Design review of the part built by this model. Coordinates are the model's own, in mm. A direction names the side the tool comes from. Coordinates: 2 decimals unless noted, no trailing zeros. Loops run counter-clockwise (first coordinate to the right, second up) from the corner with the lowest first, then second, coordinate; pieces in that order, holes last. Notation, with made-up numbers: (2.25, 28.25) - (51.25, 28.25) arc R10 cw to (51.25, 35.25) - close; hole circle Ø7 at (-19, 14.5). An arc over 180 degrees is marked (long way). Answer in a Markdown table with one row per item. Add a question column.
(1) To check wall thickness, follow L1, parallel to X at y = 41, z = 57.5; L2, parallel to X at y = 41, z = 78; L3, parallel to Y at x = 43.5, z = 97. State the ranges of each line that lie inside material, in increasing order. Write a range as [from, to].
(2) For faces 1 (the face through (57, 67, 85)), 2 (the face through (-43.325, 47.12, 64.65)), 3 (the face through (-53, -3, 90)), 4 (the face through (21, 75, 82)), list the 3-axis set-ups (+Z, -Z, +X, -X, +Y, -Y) from which the entire face can be reached by the end or side of a thin tool; tool diameter is ignored.
(3) We need section B-B, the plane x = -25.5. Write out the cut boundary in (y, z).
(4) Clearance check with flat-ended pins moving along their axes: pin 1 (9 mm diameter, centred on y = -81, z = 81.5, fed in from +X); pin 2 (10 mm diameter, centred on x = 21.5, y = -54, fed in from +Z); pin 3 (14.5 mm diameter, centred on x = -46.5, y = 39.5, fed in from +Z). State where each tip first meets the part, or that it passes through.
(5) We need section D-D, the plane z = 96.5. Write out the cut boundary in (x, y).
(6) We need section A-A, the plane y = 41. Write out the cut boundary in (x, z).
(7) We need section C-C, the plane z = 65. Write out the cut boundary in (x, y).
(8) The part is to be moulded in two halves that separate along X. For faces 5 (the face through (42, -78, 30)), 6 (the face through (-6, 100, 54)), 7 (the face through (14.566, 67.605, 89.002)), say which applies: released by +X, released by -X, zero draft, split by the parting line, or undercut.
Autodesk Fusion 360 part; units mm, degrees
sketch "Sketch1" plane through (0, 0, 0) normal (0, 0, 1) x (1, 0, 0)
  line L0 (-75, 100) -> (65, 100)
  line L1 (65, 100) -> (65, -100)
  line L2 (65, -100) -> (-75, -100)
  line L3 (-75, -100) -> (-75, 100)
  line L4 (38.9966, -100) -> (40, -100)
  line L5 (20, -100) -> (65, -55)
  line L6 (-60, -100) -> (-60, -50)
  line L7 (-60, -50) -> (-20, 30)
  line L8 (-20, 30) -> (-20, 60)
  line L9 (-20, 60) -> (50, 60)
  line L10 (50, 60) -> (70, 80)
  line L11 (70, 80) -> (70, 100)
  line L12 (-20, 60) -> (-75, 60)
extrude "Extrude1" add sketch "Sketch1" along normal blind 20 contours L1 L2 L5 L6 L7 L8 L9 L10
extrude "Extrude2" add sketch "Sketch1" along normal blind 40 contours L2 L3 L6 L7 L8 L12
extrude "Extrude3" add sketch "Sketch1" along normal blind 70 contours L0 L1 L3 L9 L10 L12
sketch "Sketch2" plane through (0, 0, 40) normal (0, 0, 1) x (-1, 0, 0)
  line L0 (60, 100) -> (60, 50)
  line L1 (60, 50) -> (20, -30)
  line L2 (20, -30) -> (20, -60)
  line L3 (20, -60) -> (75, -60)
  line L4 (75, -60) -> (75, 100)
  line L5 (75, 100) -> (60, 100)
  circle A0 centre (50, -41) radius 9.056
sketch "Sketch3" plane through (0, 60, 0) normal (0, -1, 0) x (1, 0, 0)
  line L0 (-75, 40) -> (-20, 40)
  line L1 (-20, 40) -> (-20, 20)
  line L2 (-20, 20) -> (50, 20)
  line L3 (50, 20) -> (50, 70)
  line L4 (50, 70) -> (-75, 70)
  line L5 (-75, 70) -> (-75, 40)
  circle A0 centre (20, 45) radius 11.8346
extrude "Extrude4" add 1 faces at (-5, -25, 20) along direction (0, 0, 1) blind 40
extrude "Extrude5" add sketch "Sketch2" along normal blind 50
extrude "Extrude6" add 1 faces at (-10, 86.6667, 70) along direction (0, 0, 1) blind 40
sketch "Sketch4" plane through (0, 60, 0) normal (0, -1, 0) x (1, 0, 0)
  line L0 (-20, 90) -> (-20, 60)
  line L1 (-20, 60) -> (50, 60)
  line L2 (50, 60) -> (50, 110)
  line L3 (50, 110) -> (-75, 110)
  line L4 (-75, 110) -> (-75, 90)
  line L5 (-75, 90) -> (-20, 90)
hole "Hole1" at (21.3246, 60, 81.6312) direction (0, 1, 0) diameter 20 depth 15 tip angle 180
sketch "Sketch5" plane through (0, 0, 0) normal (0, 0, 1) x (1, 0, 0)
Responses:
| question | item | result |
|---|---|---|
| 1 | L1 | x = [-75, -59.06], [-40.94, 65] |
| 1 | L2 | x = [-75, -59.06], [-40.94, -20] |
| 1 | L3 | y = [60, 100] |
| 2 | face 1 | +Z, +X, -Y |
| 2 | face 2 | +Z |
| 2 | face 3 | +Z, +X, -X, -Y |
| 2 | face 4 | -Y |
| 3 | outline | (-100, 0) - (100, 0) - (100, 110) - (60, 110) - (60, 90) - (19, 90) - (19, 60) - (-100, 60) - close |
| 4 | pin 1 | stops at x = -60 |
| 4 | pin 2 | stops at z = 60 |
| 4 | pin 3 | stops at z = 90 |
| 5 | outline | (-75, 60) - (50, 60) - (65, 75) - (65, 100) - (-75, 100) - close |
| 6 | outline | (-75, 0) - (65, 0) - (65, 60) - (-20, 60) - (-20, 90) - (-40.94, 90) - (-40.94, 40) - (-59.06, 40) - (-59.06, 90) - (-75, 90) - close |
| 7 | outline | (-75, -100) - (-60, -100) - (-60, -50) - (-20, 30) - (-20, 60) - (50, 60) - (65, 75) - (65, 100) - (-75, 100) - close; hole circle Ø18.11 at (-50, 41) |
| 8 | face 5 | released by +X |
| 8 | face 6 | zero draft |
| 8 | face 7 | undercut |
